from build123d import *

# Parameters (mm, degrees)
SKETCH1_W           = 55.5
SKETCH1_H           = 72
BOSS_EXTRUDE1_DEPTH = 12.5
SKETCH2_W           = 53
SKETCH2_H           = 61
CUT_EXTRUDE1_DEPTH  = 1.65
SKETCH3_W           = 44
SKETCH3_H           = 63.5
CUT_EXTRUDE2_DEPTH  = 11.5
SKETCH4_W           = 44
SKETCH4_H           = 4
BOSS_EXTRUDE2_DEPTH = 6.5
SKETCH5_W           = 44
SKETCH5_H           = 3.5
BOSS_EXTRUDE3_DEPTH = 3
SKETCH6_W           = 1.5
SKETCH6_H           = 56
CUT_EXTRUDE3_DEPTH  = 3
SKETCH7_W           = 7
SKETCH7_H           = 8.5
CUT_EXTRUDE4_DEPTH  = 4.5
SKETCH8_W           = 36
SKETCH8_H           = 7
CUT_EXTRUDE5_DEPTH  = 7.6
SKETCH9_W           = 39.25
SKETCH9_H           = 3.9
CUT_EXTRUDE6_DEPTH  = 6
FILLET2_R           = 2
FILLET3_R           = 1
SKETCH10_R          = 1
CUT_EXTRUDE7_DEPTH  = 48.14140961


with BuildPart() as part:
    # Sketch1 → Boss-Extrude1 (new body)
    with BuildSketch(Plane(origin=(0, 0, 0), x_dir=(1, 0, 0), z_dir=(0, 1, 0))):
        Rectangle(SKETCH1_W, SKETCH1_H)
    extrude(amount=BOSS_EXTRUDE1_DEPTH)

    # Sketch2 → Cut-Extrude1 (cut)
    with BuildSketch(Plane(origin=(0, 12.5, 0), x_dir=(1, 0, 0), z_dir=(0, 1, 0))):
        Rectangle(SKETCH2_W, SKETCH2_H)
    extrude(amount=-CUT_EXTRUDE1_DEPTH, mode=Mode.SUBTRACT)

    # Sketch3 → Cut-Extrude2 (cut)
    with BuildSketch(Plane(origin=(0, 12.5, 0), x_dir=(1, 0, 0), z_dir=(0, 1, 0))):
        with Locations((0, -2.75)):
            Rectangle(SKETCH3_W, SKETCH3_H)
    extrude(amount=-CUT_EXTRUDE2_DEPTH, mode=Mode.SUBTRACT)

    # Sketch4 → Boss-Extrude2 (add)
    with BuildSketch(Plane(origin=(0, 12.5, 0), x_dir=(1, 0, 0), z_dir=(0, 1, 0))):
        with Locations((0, -32.5)):
            Rectangle(SKETCH4_W, SKETCH4_H)
    extrude(amount=-BOSS_EXTRUDE2_DEPTH)

    # Sketch5 → Boss-Extrude3 (add)
    with BuildSketch(Plane(origin=(0, 10.85, 0), x_dir=(1, 0, 0), z_dir=(0, 1, 0))):
        with Locations((0, -28.75)):
            Rectangle(SKETCH5_W, SKETCH5_H)
    extrude(amount=-BOSS_EXTRUDE3_DEPTH)

    # Sketch6 → Cut-Extrude3 (cut)
    with BuildSketch(Plane(origin=(0, 10.85, 0), x_dir=(1, 0, 0), z_dir=(0, 1, 0))):
        with Locations((22.75, 1)):
            Rectangle(SKETCH6_W, SKETCH6_H)
        with Locations((-22.75, 1)):
            Rectangle(SKETCH6_W, SKETCH6_H)
    extrude(amount=-CUT_EXTRUDE3_DEPTH, mode=Mode.SUBTRACT)

    # Sketch7 → Cut-Extrude4 (cut)
    with BuildSketch(Plane(origin=(0, 12.5, 0), x_dir=(1, 0, 0), z_dir=(0, 1, 0))):
        with Locations((-24.25, 23)):
            Rectangle(SKETCH7_W, SKETCH7_H)
    extrude(amount=-CUT_EXTRUDE4_DEPTH, mode=Mode.SUBTRACT)

    # Sketch8 → Cut-Extrude5 (cut)
    with BuildSketch(Plane(origin=(0, 12.5, 0), x_dir=(1, 0, 0), z_dir=(0, 1, 0))):
        with Locations((6.5, 31.5)):
            Rectangle(SKETCH8_W, SKETCH8_H)
    extrude(amount=-CUT_EXTRUDE5_DEPTH, mode=Mode.SUBTRACT)

    # Sketch9 → Cut-Extrude6 (cut)
    with BuildSketch(Plane(origin=(0, 0, -36), x_dir=(-1, 0, 0), z_dir=(0, 0, -1))):
        with Locations((-8.125, 1.95)):
            Rectangle(SKETCH9_W, SKETCH9_H)
    extrude(amount=-CUT_EXTRUDE6_DEPTH, mode=Mode.SUBTRACT)

    # Fillet2
    fillet2_edges = [part.edges().sort_by_distance(p)[0] for p in [
        (-19.625, 0, -36),
        (27.75, 0, 3),
        (0, 0, 36),
        (-27.75, 0, 0),
        (27.75, 8.2, -36),
        (27.75, 6.25, 36),
        (-27.75, 6.25, 36),
    ]]
    fillet(fillet2_edges, radius=FILLET2_R)

    # Fillet3
    fillet3_edges = [part.edges().sort_by_distance(p)[0] for p in [
        (27.75, 2.95, -30),
        (27.75, 3.9, -32),
        (-11.5, 0, -32),
        (7.125, 3.9, -36),
        (-11.5, 2.95, -36),
        (7.125, 0, -30),
        (-11.5, 0.585786438, -35.414213562),
        (27.164213562, 0.585786438, -30),
        (27.164213562, 3.9, -35.414213562),
    ]]
    fillet(fillet3_edges, radius=FILLET3_R)

    # Sketch10 → Cut-Extrude7 (cut, through all)
    with BuildSketch(Plane(origin=(0, 12.5, 0), x_dir=(1, 0, 0), z_dir=(0, 1, 0))):
        with Locations(Location((24.95, -33.2, 0), (0, 0, 270))):
            Circle(SKETCH10_R)
    extrude(amount=-CUT_EXTRUDE7_DEPTH, mode=Mode.SUBTRACT)


solid = part.part
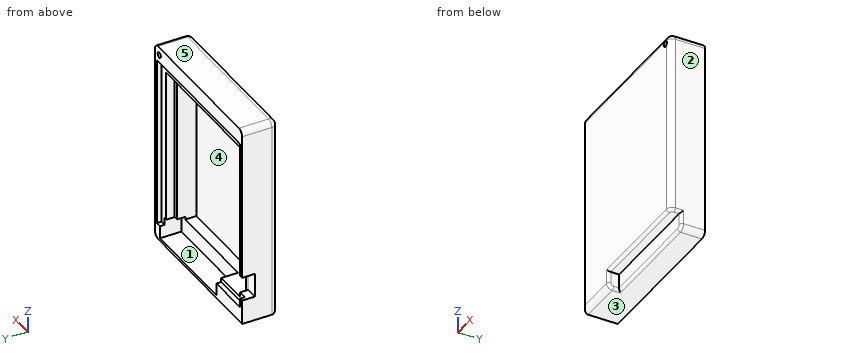
Geometry check sheet. Reference: the model listing, model coordinates, mm. Face numbers are marked on the shaded views. A direction names the side the tool comes from. Coordinates: 2 decimals unless noted, no trailing zeros. Order: outer loops, then holes, each group sorted by start corner. A loop starts at its lowest first (then second) coordinate and runs counter-clockwise, first axis right, second up. Notation, with made-up numbers: (15, 46.25) -> (70, 46.25) arc R6 ccw to (70, 57.25) -> close; hole circle Ø4 at (82, 58.5). An arc over 180 degrees is marked (long way). Use a Markdown table: item, result. Add a question column.
1. Go/stop test with flat-tipped pins: pin 1 Ø4.5 at (x, z) = (-25.5, -23) entering from +Y; pin 2 Ø2.5 at (x, z) = (7.5, -33) entering from -Y; pin 3 Ø1.2 at (x, z) = (24.95, 33.2) entering from -Y; pin 4 Ø1 at (x, z) = (-15.5, -20.5) entering from +Y. Record where each tip stops, or that it passes through.
2. Cross-section at C-C (x = -1.5). Enter the section's corners in (y, z).
3. Cross-section at A-A (x = -21). Enter the section's corners in (y, z).
4. Set-up check for the marked faces 1 and 2: record each of +Z, -Z, +X, -X, +Y, -Y from which the full face is reachable in a straight line by a thin tool's end or side.
5. Material ranges on L1, parallel to X at y = 3.5, z = 33.2; L2, parallel to Z at x = 24.95, y = 3; L3, parallel to Z at x = 24.95, y = 9, recorded low to high.
6. Mould release check, pull along Z, two halves, no side actions. Record for the marked faces 3, 4 and 5: pulls with the +Z half, pulls with the -Z half, needs draft (parallel to the pull), parting line crosses it, or undercut.
7. Cross-section at B-B (z = -7.5). Enter the section's corners in (x, y).
Filled sheet:
| question | item | result |
|---|---|---|
| 1 | pin 1 | y = 8 |
| 1 | pin 2 | y = 3.9 |
| 1 | pin 3 | through |
| 1 | pin 4 | y = 1 |
| 2 | outline | (0, -29) arc R1 ccw to (1, -30) -> (3.9, -30) -> (3.9, -35) arc R1 ccw to (4.9, -36) -> (12.5, -36) -> (12.5, -35) -> (4.9, -35) -> (4.9, -29) -> (1, -29) -> (1, 34.5) -> (6, 34.5) -> (6, 30.5) -> (7.85, 30.5) -> (7.85, 27) -> (10.85, 27) -> (10.85, 30.5) -> (12.5, 30.5) -> (12.5, 36) -> (2, 36) arc R2 ccw to (0, 34) -> close |
| 3 | outline | (0, -34) arc R2 ccw to (2, -36) -> (12.5, -36) -> (12.5, -30.5) -> (10.85, -30.5) -> (10.85, -29) -> (1, -29) -> (1, 34.5) -> (6, 34.5) -> (6, 30.5) -> (7.85, 30.5) -> (7.85, 27) -> (10.85, 27) -> (10.85, 30.5) -> (12.5, 30.5) -> (12.5, 36) -> (2, 36) arc R2 ccw to (0, 34) -> close |
| 4 | face 1 | +Y |
| 4 | face 2 | +Z, -Z, +X, +Y, -Y |
| 5 | L1 | -27.75 to -22, 22 to 23.95, 25.95 to 27.75 |
| 5 | L2 | -30 to 32.2, 34.2 to 36 |
| 5 | L3 | -36 to 32.2, 34.2 to 36 |
| 6 | face 3 | pulls with the -Z half |
| 6 | face 4 | undercut |
| 6 | face 5 | pulls with the +Z half |
| 7 | outline | (-27.75, 2) arc R2 ccw to (-25.75, 0) -> (25.75, 0) arc R2 ccw to (27.75, 2) -> (27.75, 12.5) -> (26.5, 12.5) -> (26.5, 10.85) -> (23.5, 10.85) -> (23.5, 7.85) -> (22, 7.85) -> (22, 1) -> (-22, 1) -> (-22, 7.85) -> (-23.5, 7.85) -> (-23.5, 10.85) -> (-26.5, 10.85) -> (-26.5, 12.5) -> (-27.75, 12.5) -> close |
